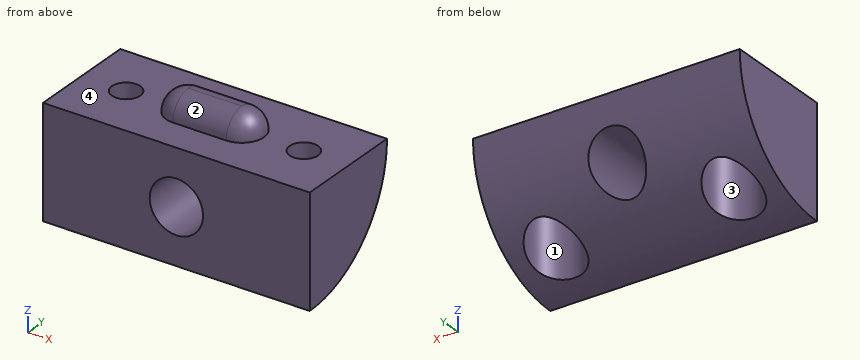
```python
from build123d import *

# Parameters (mm, degrees)
SALIENTE_EXTRUIR1_DEPTH    = 70
CORTAR_EXTRUIR1_REACH      = 74.198
CORTAR_EXTRUIR1_END_RADIUS = 12.5
CROQUIS2_R                 = 1.6
CORTAR_EXTRUIR2_REACH      = 73.614
CORTAR_EXTRUIR2_END_RADIUS = 12.5
CROQUIS3_R                 = 3
CORTAR_EXTRUIR3_REACH      = 74.198
CORTAR_EXTRUIR3_END_RADIUS = 12.5
CROQUIS4_R                 = 3
CROQUIS6_W                 = 16.861787602
CROQUIS6_H                 = 17.380881654
CORTAR_EXTRUIR5_DEPTH      = 40
SALIENTE_EXTRUIR2_DEPTH    = 2.5
REDONDEO1_R                = 2.5


with BuildPart() as part:
    # Croquis1 → Saliente-Extruir1 (new body)
    with BuildSketch(Plane(origin=(0, 0, 0), x_dir=(0, 0, -1), z_dir=(1, 0, 0))):
        with BuildLine():
            Line((0, 0), (0, 12.5))
            ThreePointArc((0, 12.5), (8.838834765, 8.838834765), (12.5, 0))
            Line((12.5, 0), (0, 0))
        make_face()
    extrude(amount=SALIENTE_EXTRUIR1_DEPTH)

    # Cortar-Extruir1: up to this cylinder (the profile starts inside it)
    cortar_extruir1_end = Plane(origin=(35, 0, 0), z_dir=(-1, 0, 0)) * Cylinder(CORTAR_EXTRUIR1_END_RADIUS, 234.396, mode=Mode.PRIVATE)
    # Croquis2 → Cortar-Extruir1 (cut, up to the surface)
    with BuildSketch(Plane.XY, mode=Mode.PRIVATE) as cortar_extruir1_sk1:
        with Locations((5, 6.25)):
            Circle(CROQUIS2_R)
    cortar_extruir1_tool1 = extrude(cortar_extruir1_sk1.sketch, amount=-CORTAR_EXTRUIR1_REACH, mode=Mode.PRIVATE) & cortar_extruir1_end
    add(cortar_extruir1_tool1.solids().sort_by_distance((5, 6.25, 0))[0], mode=Mode.SUBTRACT)
    # Croquis2 → Cortar-Extruir1 (cut, up to the surface)
    with BuildSketch(Plane.XY, mode=Mode.PRIVATE) as cortar_extruir1_sk2:
        with Locations((25, 6.25)):
            Circle(CROQUIS2_R)
    cortar_extruir1_tool2 = extrude(cortar_extruir1_sk2.sketch, amount=-CORTAR_EXTRUIR1_REACH, mode=Mode.PRIVATE) & cortar_extruir1_end
    add(cortar_extruir1_tool2.solids().sort_by_distance((25, 6.25, 0))[0], mode=Mode.SUBTRACT)
    # Croquis2 → Cortar-Extruir1 (cut, up to the surface)
    with BuildSketch(Plane.XY, mode=Mode.PRIVATE) as cortar_extruir1_sk3:
        with Locations((45, 6.25)):
            Circle(CROQUIS2_R)
    cortar_extruir1_tool3 = extrude(cortar_extruir1_sk3.sketch, amount=-CORTAR_EXTRUIR1_REACH, mode=Mode.PRIVATE) & cortar_extruir1_end
    add(cortar_extruir1_tool3.solids().sort_by_distance((45, 6.25, 0))[0], mode=Mode.SUBTRACT)
    # Croquis2 → Cortar-Extruir1 (cut, up to the surface)
    with BuildSketch(Plane.XY, mode=Mode.PRIVATE) as cortar_extruir1_sk4:
        with Locations((65, 6.25)):
            Circle(CROQUIS2_R)
    cortar_extruir1_tool4 = extrude(cortar_extruir1_sk4.sketch, amount=-CORTAR_EXTRUIR1_REACH, mode=Mode.PRIVATE) & cortar_extruir1_end
    add(cortar_extruir1_tool4.solids().sort_by_distance((65, 6.25, 0))[0], mode=Mode.SUBTRACT)

    # Cortar-Extruir2: up to this cylinder (the profile starts inside it)
    cortar_extruir2_end = Plane(origin=(35, 0, 0), z_dir=(-1, 0, 0)) * Cylinder(CORTAR_EXTRUIR2_END_RADIUS, 233.228, mode=Mode.PRIVATE)
    # Croquis3 → Cortar-Extruir2 (cut, up to the surface)
    with BuildSketch(Plane.XY.offset(-4), mode=Mode.PRIVATE) as cortar_extruir2_sk1:
        with Locations((5, 6.25)):
            Circle(CROQUIS3_R)
    cortar_extruir2_tool1 = extrude(cortar_extruir2_sk1.sketch, amount=-CORTAR_EXTRUIR2_REACH, mode=Mode.PRIVATE) & cortar_extruir2_end
    add(cortar_extruir2_tool1.solids().sort_by_distance((5, 6.25, -4))[0], mode=Mode.SUBTRACT)
    # Croquis3 → Cortar-Extruir2 (cut, up to the surface)
    with BuildSketch(Plane.XY.offset(-4), mode=Mode.PRIVATE) as cortar_extruir2_sk2:
        with Locations((25, 6.25)):
            Circle(CROQUIS3_R)
    cortar_extruir2_tool2 = extrude(cortar_extruir2_sk2.sketch, amount=-CORTAR_EXTRUIR2_REACH, mode=Mode.PRIVATE) & cortar_extruir2_end
    add(cortar_extruir2_tool2.solids().sort_by_distance((25, 6.25, -4))[0], mode=Mode.SUBTRACT)
    # Croquis3 → Cortar-Extruir2 (cut, up to the surface)
    with BuildSketch(Plane.XY.offset(-4), mode=Mode.PRIVATE) as cortar_extruir2_sk3:
        with Locations((45, 6.25)):
            Circle(CROQUIS3_R)
    cortar_extruir2_tool3 = extrude(cortar_extruir2_sk3.sketch, amount=-CORTAR_EXTRUIR2_REACH, mode=Mode.PRIVATE) & cortar_extruir2_end
    add(cortar_extruir2_tool3.solids().sort_by_distance((45, 6.25, -4))[0], mode=Mode.SUBTRACT)
    # Croquis3 → Cortar-Extruir2 (cut, up to the surface)
    with BuildSketch(Plane.XY.offset(-4), mode=Mode.PRIVATE) as cortar_extruir2_sk4:
        with Locations((65, 6.25)):
            Circle(CROQUIS3_R)
    cortar_extruir2_tool4 = extrude(cortar_extruir2_sk4.sketch, amount=-CORTAR_EXTRUIR2_REACH, mode=Mode.PRIVATE) & cortar_extruir2_end
    add(cortar_extruir2_tool4.solids().sort_by_distance((65, 6.25, -4))[0], mode=Mode.SUBTRACT)

    # Cortar-Extruir3: up to this cylinder (the profile starts inside it)
    cortar_extruir3_end = Plane(origin=(35, 0, 0), z_dir=(-1, 0, 0)) * Cylinder(CORTAR_EXTRUIR3_END_RADIUS, 214.396, mode=Mode.PRIVATE)
    # Croquis4 → Cortar-Extruir3 (cut, up to the surface)
    with BuildSketch(Plane.XZ, mode=Mode.PRIVATE) as cortar_extruir3_sk1:
        with Locations(Location((55, -6.25, 0), (0, 0, 270))):
            Circle(CROQUIS4_R)
    cortar_extruir3_tool1 = extrude(cortar_extruir3_sk1.sketch, amount=-CORTAR_EXTRUIR3_REACH, mode=Mode.PRIVATE) & cortar_extruir3_end
    add(cortar_extruir3_tool1.solids().sort_by_distance((55, 0, -6.25))[0], mode=Mode.SUBTRACT)
    # Croquis4 → Cortar-Extruir3 (cut, up to the surface)
    with BuildSketch(Plane.XZ, mode=Mode.PRIVATE) as cortar_extruir3_sk2:
        with Locations(Location((35, -6.25, 0), (0, 0, 270))):
            Circle(CROQUIS4_R)
    cortar_extruir3_tool2 = extrude(cortar_extruir3_sk2.sketch, amount=-CORTAR_EXTRUIR3_REACH, mode=Mode.PRIVATE) & cortar_extruir3_end
    add(cortar_extruir3_tool2.solids().sort_by_distance((35, 0, -6.25))[0], mode=Mode.SUBTRACT)
    # Croquis4 → Cortar-Extruir3 (cut, up to the surface)
    with BuildSketch(Plane.XZ, mode=Mode.PRIVATE) as cortar_extruir3_sk3:
        with Locations(Location((15, -6.25, 0), (0, 0, 270))):
            Circle(CROQUIS4_R)
    cortar_extruir3_tool3 = extrude(cortar_extruir3_sk3.sketch, amount=-CORTAR_EXTRUIR3_REACH, mode=Mode.PRIVATE) & cortar_extruir3_end
    add(cortar_extruir3_tool3.solids().sort_by_distance((15, 0, -6.25))[0], mode=Mode.SUBTRACT)

    # Croquis6 → Cortar-Extruir5 (cut)
    with BuildSketch(Plane.ZY):
        with Locations((-8.430893801, 8.690440827)):
            Rectangle(CROQUIS6_W, CROQUIS6_H)
    extrude(amount=-CORTAR_EXTRUIR5_DEPTH, mode=Mode.SUBTRACT)

    # Croquis7 → Saliente-Extruir2 (add)
    with BuildSketch(Plane.XY):
        with BuildLine():
            Line((58, 8.75), (52, 8.75))
            ThreePointArc((52, 8.75), (49.5, 6.25), (52, 3.75))
            Line((52, 3.75), (58, 3.75))
            ThreePointArc((58, 3.75), (60.5, 6.25), (58, 8.75))
        make_face()
    extrude(amount=SALIENTE_EXTRUIR2_DEPTH)

    # Redondeo1
    redondeo1_edges = [part.edges().sort_by_distance(p)[0] for p in [
        (55, 3.75, 2.5),
        (49.5, 6.25, 2.5),
        (55, 8.75, 2.5),
        (60.5, 6.25, 2.5),
    ]]
    fillet(redondeo1_edges, radius=REDONDEO1_R - 0.0001)  # a hair under: the kernel refuses the full size


solid = part.part
```
Here's how the part is built. I have some questions about the finished solid (model axes, mm). Face numbers are marked on the shaded views. Coordinates: 2 decimals unless noted, no trailing zeros. Loops run counter-clockwise (first coordinate to the right, second up) from the corner with the lowest first, then second, coordinate; pieces in that order, holes last. Notation, with made-up numbers: (24, -28) - (41, -28) arc R11 cw to (41, -22) - close; hole circle Ø5 at (36, 85.25). An arc over 180 degrees is marked (long way). Return JSON: item names as keys, results as strings. Group by question number.
Item 1: I need wall thicknesses on line 1 (X direction, y = 8.5, z = -9); line 2 (Y direction, x = 67.5, z = -8.75); line 3 (Y direction, x = 45, z = -2). Which ranges of each line are inside material? Lowest first, please. Write a range as from..to.
Item 2: If we section it at D-D on x = 63: Write out the boundary of the cut face in (y, z).
Item 3: Will these pins go through, and if not, where does the flat tip stop? P1, Ø3, axis at x = 45.5, y = 3, coming from the +Z side; P2, Ø3.5, axis at x = 65, y = 6.25, coming from the -Z side; P3, Ø6.5, axis at x = 65.5, y = 5.5, coming from the -Z side.
Item 4: We'd pull the mould along Y, two halves only. Please class the marked faces 1, 2, 3 and 4: +Y half, -Y half, draft (parallel to the pull), parting line (faces both ways), or undercut.
Item 5: If we section it at A-A on z = -7.75: Write out the boundary of the cut face in (x, y).
Item 6: If we section it at C-C on y = 2.25: Write out the boundary of the cut face in (x, z), and give its area (3 significant figures).
Calculated:
{
 "1": {"line 1": "x = 40..43.02, 46.98..53.8, 56.2..63.02, 66.98..70", "line 2": "y = 0..4.59, 7.91..8.93", "line 3": "y = 0..4.65, 7.85..12.34"},
 "2": {"outline": "(0, -12.5) arc R12.5 ccw to (4.01, -11.84) - (4.01, -4) - (8.49, -4) - (8.49, -9.18) arc R12.5 ccw to (12.5, 0) - (0, 0) - close"},
 "3": {"P1": "stops at z = 0", "P2": "stops at z = -4", "P3": "stops at z = -12.3"},
 "4": {"face 1": "undercut", "face 2": "-Y half", "face 3": "undercut", "face 4": "draft"},
 "5": {"outline": "(40, 0) - (52.4, 0) - (52.4, 9.81) - (40, 9.81) - close; (57.6, 0) - (70, 0) - (70, 9.81) - (57.6, 9.81) - close; hole circle Ø6 at (45, 6.25); hole circle Ø6 at (65, 6.25)"},
 "6": {"outline": "(40, -12.3) - (70, -12.3) - (70, 0) - (40, 0) - close; hole circle Ø6 at (55, -6.25)", "area": "341 mm^2"}
}
